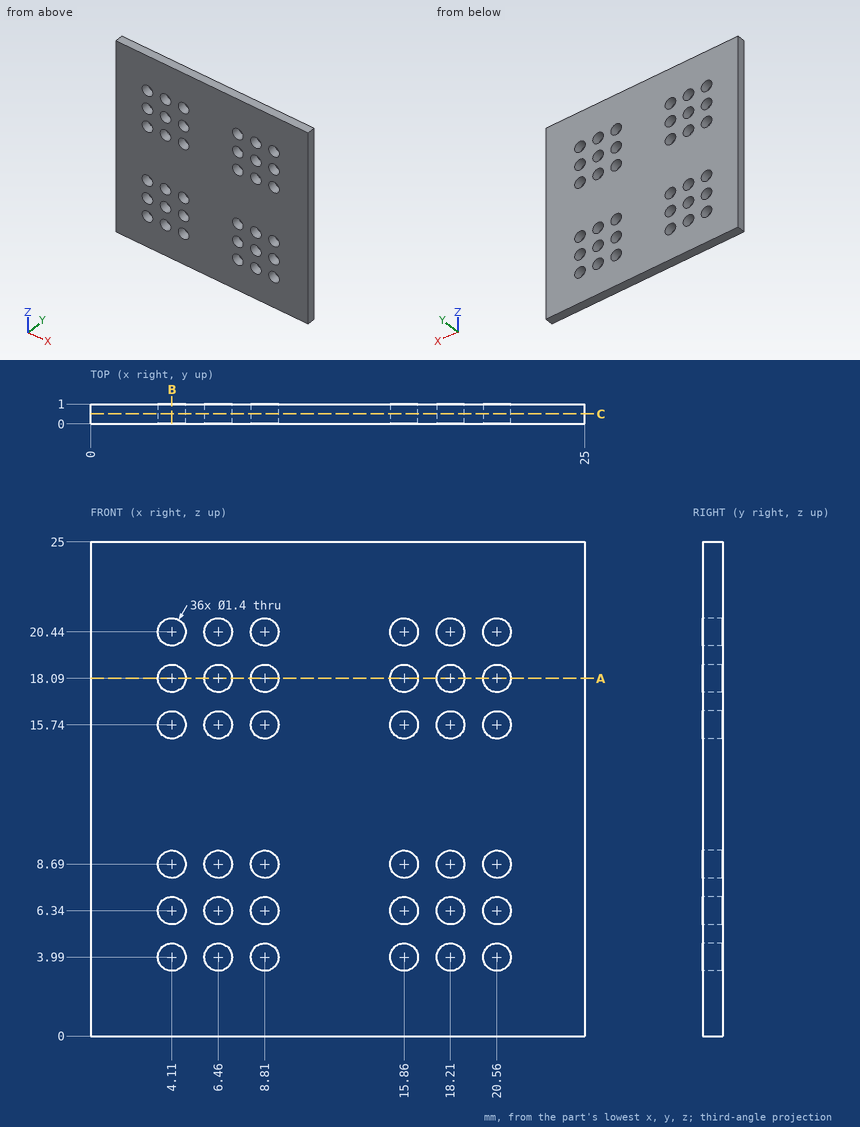
Study the drawing (mm; zero at the part's minimum x, y, z) and answer. Coordinates: 2 decimals unless noted, no trailing zeros. Write each loop counter-clockwise with the first axis right and the second up, starting at its lowest first coordinate (ties: lowest second). Pieces come first, ordered by that corner, then holes.
Q1. A cutting plane is placed at C-C, the plane y = 0.5. State how many separate pieces and enclosed holes the cut face has, then the cut area to 3 significant figures.
Q2. This flat-tipped pin is pushed along its axis until it touches: pin 1 Ø1.1 at (x, z) = (8.81, 8.69) entering from +Y. Where does it stop, or does it pass through?
Q3. A cutting plane is placed at A-A, the plane z = 18.09. Give the vertices of the cut face in (x, y), then the cut area to 3 significant figures.
Q4. A cutting plane is placed at B-B, the plane x = 4.11. Give the vertices of the cut face in (y, z).
Findings below:
1. separate pieces: 1
1. enclosed holes: 36
1. area: 570 mm2
2. pin 1: passes through
3. outline: (0, 0) - (3.41, 0) - (3.41, 1) - (0, 1) - close; (4.81, 0) - (5.76, 0) - (5.76, 1) - (4.81, 1) - close; (7.16, 0) - (8.11, 0) - (8.11, 1) - (7.16, 1) - close; (9.51, 0) - (15.16, 0) - (15.16, 1) - (9.51, 1) - close; (16.56, 0) - (17.51, 0) - (17.51, 1) - (16.56, 1) - close; (18.91, 0) - (19.86, 0) - (19.86, 1) - (18.91, 1) - close; (21.26, 0) - (25, 0) - (25, 1) - (21.26, 1) - close
3. area: 16.6 mm2
4. outline: (0, 0) - (1, 0) - (1, 3.29) - (0, 3.29) - close; (0, 4.69) - (1, 4.69) - (1, 5.64) - (0, 5.64) - close; (0, 7.04) - (1, 7.04) - (1, 7.99) - (0, 7.99) - close; (0, 9.39) - (1, 9.39) - (1, 15.04) - (0, 15.04) - close; (0, 16.44) - (1, 16.44) - (1, 17.39) - (0, 17.39) - close; (0, 18.79) - (1, 18.79) - (1, 19.74) - (0, 19.74) - close; (0, 21.14) - (1, 21.14) - (1, 25) - (0, 25) - close
